from build123d import *

# Parameters (mm, degrees)
SKETCH1_W           = 23
SKETCH1_H           = 65
BOSS_EXTRUDE1_DEPTH = 66
SKETCH2_W           = 60
SKETCH2_H           = 17
CUT_EXTRUDE1_DEPTH  = 66
CUT_EXTRUDE2_REACH  = 25
SKETCH3_W           = 32
SKETCH3_H           = 53
CUT_EXTRUDE3_REACH  = 25
SKETCH5_R           = 4.5
SKETCH5_R_2         = 2.530586218
SKETCH5_R_3         = 2.69284222
SKETCH6_W           = 17
SKETCH6_H           = 15
CUT_EXTRUDE4_DEPTH  = 20


with BuildPart() as part:
    # Sketch1 → Boss-Extrude1 (new body)
    with BuildSketch(Plane(origin=(0, 0, 0), x_dir=(0, 0, -1), z_dir=(1, 0, 0))):
        with Locations((-11.5, -32.5)):
            Rectangle(SKETCH1_W, SKETCH1_H)
    extrude(amount=-BOSS_EXTRUDE1_DEPTH)

    # Sketch2 → Cut-Extrude1 (cut, through all)
    with BuildSketch(Plane(origin=(0, 0, 0), x_dir=(1, 0, 0), z_dir=(0, 1, 0))):
        with Locations((-33, -11.5)):
            Rectangle(SKETCH2_W, SKETCH2_H)
    extrude(amount=-CUT_EXTRUDE1_DEPTH, mode=Mode.SUBTRACT)

    # Sketch3 → Cut-Extrude2 (cut, up to next)
    with BuildSketch(Plane.XY.offset(23), mode=Mode.PRIVATE) as cut_extrude2_sk1:
        with Locations((-33, -26.5)):
            Rectangle(SKETCH3_W, SKETCH3_H)
    cut_extrude2_tool1 = extrude(cut_extrude2_sk1.sketch, amount=-CUT_EXTRUDE2_REACH, mode=Mode.PRIVATE) & part.part
    add(cut_extrude2_tool1.solids().sort_by_distance((-33, -26.5, 23))[0], mode=Mode.SUBTRACT)

    # Sketch5 → Cut-Extrude3 (cut, up to next)
    with BuildSketch(Plane(origin=(0, 0, 0), x_dir=(-1, 0, 0), z_dir=(0, 0, -1)), mode=Mode.PRIVATE) as cut_extrude3_sk1:
        with Locations((33, -37)):
            Circle(SKETCH5_R)
    cut_extrude3_tool1 = extrude(cut_extrude3_sk1.sketch, amount=-CUT_EXTRUDE3_REACH, mode=Mode.PRIVATE) & part.part
    add(cut_extrude3_tool1.solids().sort_by_distance((-33, -37, 0))[0], mode=Mode.SUBTRACT)
    # Sketch5 → Cut-Extrude3 (cut, up to next)
    with BuildSketch(Plane(origin=(0, 0, 0), x_dir=(-1, 0, 0), z_dir=(0, 0, -1)), mode=Mode.PRIVATE) as cut_extrude3_sk2:
        with Locations((8, -7)):
            Circle(SKETCH5_R_2)
    cut_extrude3_tool2 = extrude(cut_extrude3_sk2.sketch, amount=-CUT_EXTRUDE3_REACH, mode=Mode.PRIVATE) & part.part
    add(cut_extrude3_tool2.solids().sort_by_distance((-8, -7, 0))[0], mode=Mode.SUBTRACT)
    # Sketch5 → Cut-Extrude3 (cut, up to next)
    with BuildSketch(Plane(origin=(0, 0, 0), x_dir=(-1, 0, 0), z_dir=(0, 0, -1)), mode=Mode.PRIVATE) as cut_extrude3_sk3:
        with Locations((58, -7)):
            Circle(SKETCH5_R_3)
    cut_extrude3_tool3 = extrude(cut_extrude3_sk3.sketch, amount=-CUT_EXTRUDE3_REACH, mode=Mode.PRIVATE) & part.part
    add(cut_extrude3_tool3.solids().sort_by_distance((-58, -7, 0))[0], mode=Mode.SUBTRACT)

    # Sketch6 → Cut-Extrude4 (cut)
    with BuildSketch(Plane.XY.offset(23)):
        with Locations((-57.5, -7.5)):
            Rectangle(SKETCH6_W, SKETCH6_H)
        with Locations((-8.5, -7.5)):
            Rectangle(SKETCH6_W, SKETCH6_H)
    extrude(amount=-CUT_EXTRUDE4_DEPTH, mode=Mode.SUBTRACT)


solid = part.part
Could you check a few things on this model? Use its own coordinates, in mm. A direction names the side the tool comes from. Coordinates: 2 decimals unless noted, no trailing zeros. Loops run counter-clockwise (first coordinate to the right, second up) from the corner with the lowest first, then second, coordinate; pieces in that order, holes last.
1. Imagine slicing it at A-A (y = -7). Please give me the cut outline in (x, z).
2. Imagine slicing it at C-C (x = -33). Please give me the cut outline in (y, z).
3. For faces 4 (the face through (-3, -40, 12)), 5 (the face through (-63.2, -15, 15.3)), 6 (the face through (-49, -34, 22)), which set-ups out of +Z, -Z, +X, -X, +Y, -Y let a thin tool reach every point of the face, with its end or its side?
4. Imagine slicing it at B-B (x = -26). Please give me the cut outline in (y, z), and give its area (3 significant figures).
5. For P1, Ø1.5, axis at x = -31, z = 22, coming from the +Y side; P2, Ø5, axis at x = -4.5, z = 8.5, coming from the +Y side; P3, Ø11.5, axis at x = -33, y = -37, coming from the +Z side, each with a flat end and sliding along its axis, tell me the tip position at first contact or that it passes through.
6. I need wall thicknesses on L1, parallel to Z at x = -62, y = -40; L2, parallel to X at y = -22.5, z = 14.25; L3, parallel to X at y = -38, z = 22.25. Which ranges of each line are inside material? Lowest first, please.
7. We'd pull the mould along X, two halves only. Please class faces 1 (the face through (-33, -32, 3)), 2 (the face through (-2, -15, 16)), 3 (the face through (-66, -39, 12)): released by +X, released by -X, zero draft, split by the parting line, or undercut.
8. Imagine slicing it at D-D (z = 18.5). Please give me the cut outline in (x, y), and give its area (3 significant figures).
Computed values:
1. outline: (-66, 0) - (-60.69, 0) - (-60.69, 3) - (-66, 3) - close; (-55.31, 0) - (-10.53, 0) - (-10.53, 3) - (-55.31, 3) - close; (-5.47, 0) - (0, 0) - (0, 3) - (-5.47, 3) - close
2. outline: (-65, 0) - (-41.5, 0) - (-41.5, 3) - (-65, 3) - close; (-65, 20) - (-53, 20) - (-53, 23) - (-65, 23) - close; (-32.5, 0) - (0, 0) - (0, 3) - (-32.5, 3) - close
3. face 4: +Y, -Y
3. face 5: +Z, +X, -X, +Y
3. face 6: +Z, +Y
4. outline: (-65, 0) - (0, 0) - (0, 3) - (-65, 3) - close; (-65, 20) - (-53, 20) - (-53, 23) - (-65, 23) - close
4. area: 231 mm2
5. P1: stops at y = -53
5. P2: stops at y = -15
5. P3: stops at z = 3
6. L1: z = 0 to 3, 20 to 23
6. L2: x = -66 to -63, -3 to 0
6. L3: x = -66 to -49, -17 to 0
7. face 1: undercut
7. face 2: zero draft
7. face 3: released by -X
8. outline: (-66, -65) - (-63, -65) - (-63, -15) - (-66, -15) - close; (-3, -65) - (0, -65) - (0, -15) - (-3, -15) - close
8. area: 300 mm2
